```python
from build123d import *

# Parameters (mm, degrees)
SKETCH1_R           = 18.4
BOSS_EXTRUDE1_DEPTH = 50.8
BOSS_EXTRUDE2_DEPTH = 5
FILLET1_R           = 5
SKETCH3_R           = 9
BOSS_EXTRUDE3_DEPTH = 20


with BuildPart() as part:
    # Sketch1 → Boss-Extrude1 (new body)
    with BuildSketch(Plane(origin=(0, 0, 0), x_dir=(1, 0, 0), z_dir=(0, 1, 0))):
        Circle(SKETCH1_R)
    extrude(amount=BOSS_EXTRUDE1_DEPTH)

    # Sketch2 → Boss-Extrude2 (add)
    with BuildSketch(Plane(origin=(0, 50.8, 0), x_dir=(1, 0, 0), z_dir=(0, 1, 0))):
        Polygon((0, 25), (-43.301270189, 0), (0, -25), (43.301270189, 0), align=None)
    extrude(amount=BOSS_EXTRUDE2_DEPTH)

    # Fillet1
    fillet1_edges = [part.edges().sort_by_distance(p)[0] for p in [
        (43.301270189, 53.3, 0),
        (0, 53.3, -25),
        (-43.301270189, 53.3, 0),
        (0, 53.3, 25),
    ]]
    fillet(fillet1_edges, radius=FILLET1_R)

    # Sketch3 → Boss-Extrude3 (add)
    with BuildSketch(Plane(origin=(0, 55.8, 0), x_dir=(1, 0, 0), z_dir=(0, 1, 0))):
        Circle(SKETCH3_R)
    extrude(amount=BOSS_EXTRUDE3_DEPTH)


solid = part.part
```
Design review of the part built by this model. Coordinates are the model's own, in mm. A direction names the side the tool comes from. Give positions to 0.01 mm unless a question says otherwise; leave off trailing zeros. Write each loop counter-clockwise with the first axis right and the second up, starting at its lowest first coordinate (ties: lowest second). Pieces come first, ordered by that corner, then holes. Notation, with made-up numbers: (-35.75, 31.5) - (11.25, 31.5) arc R33 cw to (11.25, 66.5) - close; hole circle Ø9 at (61, 20.5). An arc over 180 degrees is marked (long way). Return JSON: item names as keys, results as strings. Group by question number.
(1) To check wall thickness, follow probe 1 along Y at (x, z) = (8.5, -12.5); probe 2 along Y at (x, z) = (-33, -5); probe 3 along Z at (x, y) = (7.5, 11). State the ranges of each line that lie inside material, in increasing order.
(2) We need section C-C, the plane y = 52.5. Give the boundary of the cut face in (x, z), then the cut area to 3 significant figures.
(3) Insertion check: pin 1 (3 mm diameter, centred on y = 8.5, z = -3, fed in from -X); pin 2 (3 mm diameter, centred on x = 1, y = 61.5, fed in from +Z); pin 3 (1 mm diameter, centred on x = -21.5, y = 49, fed in from -Z); pin 4 (1 mm diameter, centred on x = 6, y = 29.5, fed in from +Z). Each pin has a flat end and moves straight along its axis. Give the tip position at first contact, or say it passes through.
(4) We need section B-B, the plane z = 0. Give the boundary of the cut face in (x, y).
(5) Machinability: for faces 1 (the cylindrical face through (-14.6, 25, 11.2)), 2 (the cylindrical face through (-1.172, 65.66, -8.923)), 3 (the cylindrical face through (38.3, 53.3, -0.1)), which of the approach directions +Z, -Z, +X, -X, +Y, -Y give a long, thin tool a straight path to every point of the face, cutting with its end or side? Answer none if there is none.
(6) We need section D-D, the plane x = -14. Give the boundary of the cut face in (y, z).
(7) We need section A-A, the plane x = 0. Give the boundary of the cut face in (y, z).
Reported:
{
 "1": {"probe 1": "y = 0 to 55.8", "probe 2": "y = 50.8 to 55.8", "probe 3": "z = -16.8 to 16.8"},
 "2": {"outline": "(-35.8, -4.33) - (-2.5, -23.56) arc R5 ccw to (2.5, -23.56) - (35.8, -4.33) arc R5 ccw to (35.8, 4.33) - (2.5, 23.56) arc R5 ccw to (-2.5, 23.56) - (-35.8, 4.33) arc R5 ccw to start", "area": "2,130 mm2"},
 "3": {"pin 1": "stops at x = -18.34", "pin 2": "stops at z = 9", "pin 3": "passes through", "pin 4": "stops at z = 17.56"},
 "4": {"outline": "(-38.3, 50.8) - (-18.4, 50.8) - (-18.4, 0) - (18.4, 0) - (18.4, 50.8) - (38.3, 50.8) - (38.3, 55.8) - (9, 55.8) - (9, 75.8) - (-9, 75.8) - (-9, 55.8) - (-38.3, 55.8) - close"},
 "5": {"face 1": "-Y", "face 2": "+Y", "face 3": "+X, +Y, -Y"},
 "6": {"outline": "(0, -11.94) - (50.8, -11.94) - (50.8, -16.92) - (55.8, -16.92) - (55.8, 16.92) - (50.8, 16.92) - (50.8, 11.94) - (0, 11.94) - close"},
 "7": {"outline": "(0, -18.4) - (50.8, -18.4) - (50.8, -24.23) - (55.8, -24.23) - (55.8, -9) - (75.8, -9) - (75.8, 9) - (55.8, 9) - (55.8, 24.23) - (50.8, 24.23) - (50.8, 18.4) - (0, 18.4) - close"}
}
